```python
from build123d import *

# Parameters (mm, degrees)
ESQUISSE1_W                    = 62
ESQUISSE1_H                    = 42
BOSS_EXTRU_1_DEPTH             = 3.3
ESQUISSE2_W                    = 8
ESQUISSE2_H                    = 3.3
BOSS_EXTRU_2_DEPTH             = 3.3
R_P_TITION_LIN_AIRE1_COUNT     = 2
R_P_TITION_LIN_AIRE1_PITCH     = 16
R_P_TITION_LIN_AIRE1_COL_COUNT = 2
R_P_TITION_LIN_AIRE1_COL_PITCH = 16
SYM_TRIE1_COPY_1_SKETCH_W      = 8
SYM_TRIE1_COPY_1_SKETCH_H      = 3.3
SYM_TRIE1_COPY_1_DEPTH         = 3.3
SYM_TRIE1_COPY_2_SKETCH_W      = 8
SYM_TRIE1_COPY_2_SKETCH_H      = 3.3
SYM_TRIE1_COPY_2_DEPTH         = 3.3
ESQUISSE3_W                    = 3.3
ESQUISSE3_H                    = 8
BOSS_EXTRU_3_DEPTH             = 3.3
R_P_TITION_LIN_AIRE2_COUNT     = 2
R_P_TITION_LIN_AIRE2_PITCH     = 16
R_P_TITION_LIN_AIRE2_COL_COUNT = 2
R_P_TITION_LIN_AIRE2_COL_PITCH = 16
SYM_TRIE2_COPY_1_SKETCH_W      = 3.3
SYM_TRIE2_COPY_1_SKETCH_H      = 8
SYM_TRIE2_COPY_1_DEPTH         = 3.3
SYM_TRIE2_COPY_2_SKETCH_W      = 3.3
SYM_TRIE2_COPY_2_SKETCH_H      = 8
SYM_TRIE2_COPY_2_DEPTH         = 3.3
ESQUISSE4_R                    = 4.5
ESQUISSE4_W                    = 28
ESQUISSE4_H                    = 27.5
ENL_V_MAT_EXTRU_2_DEPTH        = 1
ENL_V_MAT_EXTRU_2_DEPTH_BACK   = 4.3


with BuildPart() as part:
    # Esquisse1 → Boss.-Extru.1 (new body)
    with BuildSketch(Plane.XY):
        Rectangle(ESQUISSE1_W, ESQUISSE1_H)
    extrude(amount=BOSS_EXTRU_1_DEPTH)

    # Esquisse2 → Boss.-Extru.2 (add)
    with BuildSketch(Plane.XY.offset(3.3)):
        with Locations((0, 22.65)):
            Rectangle(ESQUISSE2_W, ESQUISSE2_H)
    boss_extru_2 = extrude(amount=-BOSS_EXTRU_2_DEPTH)

    # Répétition linéaire1: Boss.-Extru.2 ×2
    with Locations(*[(-i * R_P_TITION_LIN_AIRE1_PITCH, 0, 0) for i in range(1, R_P_TITION_LIN_AIRE1_COUNT)]):
        add(boss_extru_2)

    # Répétition linéaire1 col: Boss.-Extru.2 ×2
    with Locations(*[(i * R_P_TITION_LIN_AIRE1_COL_PITCH, 0, 0) for i in range(1, R_P_TITION_LIN_AIRE1_COL_COUNT)]):
        add(boss_extru_2)

    # Symétrie1: Boss.-Extru.2 across plane
    add(boss_extru_2.mirror(Plane.ZX))

    # Symétrie1 copy 1 sketch → Symétrie1 copy 1 (add)
    with BuildSketch(Plane(origin=(-16, 0, 3.3), x_dir=(1, 0, 0), z_dir=(0, 0, 1))):
        with Locations((0, -22.65)):
            Rectangle(SYM_TRIE1_COPY_1_SKETCH_W, SYM_TRIE1_COPY_1_SKETCH_H)
    extrude(amount=-SYM_TRIE1_COPY_1_DEPTH)

    # Symétrie1 copy 2 sketch → Symétrie1 copy 2 (add)
    with BuildSketch(Plane(origin=(16, 0, 3.3), x_dir=(1, 0, 0), z_dir=(0, 0, 1))):
        with Locations((0, -22.65)):
            Rectangle(SYM_TRIE1_COPY_2_SKETCH_W, SYM_TRIE1_COPY_2_SKETCH_H)
    extrude(amount=-SYM_TRIE1_COPY_2_DEPTH)

    # Esquisse3 → Boss.-Extru.3 (add)
    with BuildSketch(Plane.XY.offset(3.3)):
        with Locations((-32.65, 0)):
            Rectangle(ESQUISSE3_W, ESQUISSE3_H)
    boss_extru_3 = extrude(amount=-BOSS_EXTRU_3_DEPTH)

    # Répétition linéaire2: Boss.-Extru.3 ×2
    with Locations(*[(0, i * R_P_TITION_LIN_AIRE2_PITCH, 0) for i in range(1, R_P_TITION_LIN_AIRE2_COUNT)]):
        add(boss_extru_3)

    # Répétition linéaire2 col: Boss.-Extru.3 ×2
    with Locations(*[(0, -i * R_P_TITION_LIN_AIRE2_COL_PITCH, 0) for i in range(1, R_P_TITION_LIN_AIRE2_COL_COUNT)]):
        add(boss_extru_3)

    # Symétrie2: Boss.-Extru.3 across plane
    add(boss_extru_3.mirror(Plane(origin=(0, 0, 0), x_dir=(0, 0, 1), z_dir=(1, 0, 0))))

    # Symétrie2 copy 1 sketch → Symétrie2 copy 1 (add)
    with BuildSketch(Plane(origin=(0, 16, 3.3), x_dir=(-1, 0, 0), z_dir=(0, 0, 1))):
        with Locations((-32.65, 0)):
            Rectangle(SYM_TRIE2_COPY_1_SKETCH_W, SYM_TRIE2_COPY_1_SKETCH_H)
    extrude(amount=-SYM_TRIE2_COPY_1_DEPTH)

    # Symétrie2 copy 2 sketch → Symétrie2 copy 2 (add)
    with BuildSketch(Plane(origin=(0, -16, 3.3), x_dir=(-1, 0, 0), z_dir=(0, 0, 1))):
        with Locations((-32.65, 0)):
            Rectangle(SYM_TRIE2_COPY_2_SKETCH_W, SYM_TRIE2_COPY_2_SKETCH_H)
    extrude(amount=-SYM_TRIE2_COPY_2_DEPTH)

    # Esquisse4 → Enlèv. mat.-Extru.2 (cut, two sides)
    with BuildSketch(Plane(origin=(0, 0, 0), x_dir=(-1, 0, 0), z_dir=(0, 0, -1))) as enl_v_mat_extru_2_sk:
        with Locations((-18.697468538, -15.21869301)):
            Circle(ESQUISSE4_R)
        with Locations((-3.457468538, -15.21869301)):
            Circle(ESQUISSE4_R)
        with Locations((11.782531462, -15.21869301)):
            Circle(ESQUISSE4_R)
        with Locations((-0.267723221, 5.663046026)):
            Rectangle(ESQUISSE4_W, ESQUISSE4_H)
    extrude(amount=ENL_V_MAT_EXTRU_2_DEPTH, mode=Mode.SUBTRACT)
    extrude(enl_v_mat_extru_2_sk.sketch, amount=-ENL_V_MAT_EXTRU_2_DEPTH_BACK, mode=Mode.SUBTRACT)


solid = part.part
```
Read the model definition and answer for the solid it produces. Units are mm, in the model's axes. A direction names the side the tool comes from. Give positions to 0.01 mm unless a question says otherwise; leave off trailing zeros. Write each loop counter-clockwise with the first axis right and the second up, starting at its lowest first coordinate (ties: lowest second). Pieces come first, ordered by that corner, then holes. Notation, with made-up numbers: (11, -22.5) - (45, -22.5) arc R13 cw to (45, -12.5) - close; hole circle Ø10 at (-39, 48.5). An arc over 180 degrees is marked (long way). Write item = value, one per line. Start each with the question number.
Item 1: Find the intervals of material crossed by probe 1 along X at (y, z) = (-15, 0.8); probe 2 along X at (y, z) = (-3, 1.05); probe 3 along Y at (x, z) = (10.5, 1.65), in increasing order. Write a range as [from, to].
Item 2: Each of these flat-tipped pins is pushed along its axis until it touches: P1, Ø1.5, axis at x = -12.5, y = 8.5, coming from the +Z side; P2, Ø1.6, axis at y = -22, z = 2.5, coming from the -X side; P3, Ø1, axis at y = 22, z = 2.5, coming from the +X side; P4, Ø1, axis at x = -33, z = 2, coming from the +Y side. Where does it stop, or does it pass through?
Item 3: A tool of negligible diameter and unlimited length cuts with its end or side. For faces 1 (the flat face through (-33, -20, 2)), 2 (the flat face through (0, -8.087, 2)), 3 (the flat face through (33, -4, 2)), 4 (the flat face through (20, 23, 2)), from which of +Z, -Z, +X, -X, +Y, -Y can it reach the whole face along a straight path? Write none if from no direction.
Item 4: Find section A-A (y = 6.5). Give the vertices of the cut face in (x, z).
Item 5: The mould has two halves that part along Y. Classify faces 5 (the flat face through (-33, 12, 2)), 6 (the flat face through (12, -23, 2)), 7 (the cylindrical face through (14.54, -16.94, 1.63)), 8 (the flat face through (25, 21, 2)): +Y half, -Y half, draft (parallel to the pull), parting line (faces both ways), or undercut.
Item 6: Find section D-D (z = 1.7). State how many separate pieces and enclosed holes the cut face has, then the cut area to 3 significant figures.
Item 7: Find section B-B (x = 10). Give the vertices of the cut face in (y, z), then the cut area to 4 significant figures.
Item 8: Find section C-C (y = -17.5). Give the vertices of the cut face in (x, z), then the cut area to 3 significant figures.
Response:
q1.probe_1 = [-34.3, -16.28], [-7.29, -1.04], [7.95, 14.2], [23.19, 34.3]
q1.probe_2 = [-34.3, -13.73], [14.27, 34.3]
q1.probe_3 = [-21, -8.09], [19.41, 21]
q2.P1 = through
q2.P2 = -20
q2.P3 = 20
q2.P4 = 20
q3.face_1 = +Z, -Z, -X, -Y
q3.face_2 = +Z, -Z
q3.face_3 = +Z, -Z, +X
q3.face_4 = +Z, -Z, +X, +Y
q4.outline = (-31, 0) - (-13.73, 0) - (-13.73, 3.3) - (-31, 3.3) - close; (14.27, 0) - (31, 0) - (31, 3.3) - (14.27, 3.3) - close
q5.face_5 = undercut
q5.face_6 = draft
q5.face_7 = undercut
q5.face_8 = +Y half
q6.separate_pieces = 1
q6.enclosed_holes = 4
q6.area = 1,960 mm²
q7.outline = (-21, 0) - (-8.09, 0) - (-8.09, 3.3) - (-21, 3.3) - close; (19.41, 0) - (21, 0) - (21, 3.3) - (19.41, 3.3) - close
q7.area = 47.85 mm²
q8.outline = (-34.3, 0) - (-15.66, 0) - (-15.66, 3.3) - (-34.3, 3.3) - close; (-7.9, 0) - (-0.42, 0) - (-0.42, 3.3) - (-7.9, 3.3) - close; (7.34, 0) - (14.82, 0) - (14.82, 3.3) - (7.34, 3.3) - close; (22.58, 0) - (34.3, 0) - (34.3, 3.3) - (22.58, 3.3) - close
q8.area = 150 mm²
